Read the model definition and answer for the solid it produces. Units are mm, in the model's axes. Face numbers are marked on the shaded views. A direction names the side the tool comes from. Coordinates: 2 decimals unless noted, no trailing zeros. Write each loop counter-clockwise with the first axis right and the second up, starting at its lowest first coordinate (ties: lowest second). Pieces come first, ordered by that corner, then holes. Notation, with made-up numbers: (-19.75, -23.75) -> (-2.75, -23.75) arc R18 cw to (-2.75, -10.75) -> close; hole circle Ø11 at (76, -35.5). An arc over 180 degrees is marked (long way). Answer in a Markdown table with one row per item. Add a question column.
Item 1: Section C-C on z = 0.65 is taken. Write down the section's boundary in (x, y), then the cut area to 3 significant figures.
Item 2: Section A-A on y = 1.2 is taken. Write down the section's boundary in (x, z), then the cut area to 3 significant figures.
Item 3: Straight lines are drawn through the part: line 1 (X direction, y = 1.1, z = 2.4); line 2 (Z direction, x = -1.7, y = 3.7); line 3 (Z direction, x = -1.9, y = 1.4). For each, find the intervals that lie inside material, in ascending order. Write a range as from..to.
Item 4: Which of the six approach directions +Z, -Z, +X, -X, +Y, -Y give full straight-line access (tool end or side, diameter ignored) to the marked faces 1, 2 and 3?
Item 5: Section B-B on x = -1.55 is taken. Write down the section's boundary in (y, z).
Item 6: Section D-D on y = 4.4 is taken. Write down the section's boundary in (x, z), then the cut area to 3 significant figures.
```python
from build123d import *

# Parameters (mm, degrees)
SKETCH1_W           = 6
SKETCH1_H           = 6
BOSS_EXTRUDE1_DEPTH = 5
CUT_EXTRUDE1_DEPTH  = 2


with BuildPart() as part:
    # Sketch1 → Boss-Extrude1 (new body)
    with BuildSketch(Plane(origin=(0, 0, 0), x_dir=(1, 0, 0), z_dir=(0, 1, 0))):
        Rectangle(SKETCH1_W, SKETCH1_H)
    extrude(amount=BOSS_EXTRUDE1_DEPTH)

    # Sketch2 → Cut-Extrude1 (cut)
    with BuildSketch(Plane.ZY.offset(3)):
        Polygon((3, 5), (0, 5), (3, 2.5), align=None)
        Polygon((3, 0), (3, 2.5), (0, 0), align=None)
    extrude(amount=-CUT_EXTRUDE1_DEPTH, mode=Mode.SUBTRACT)


solid = part.part
```
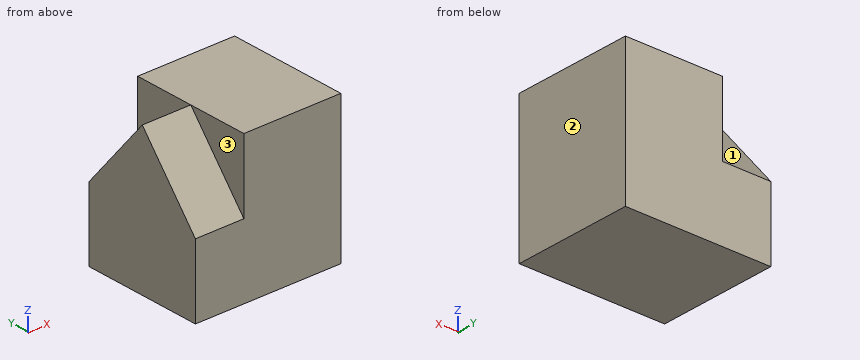
Results below:
| question | item | result |
|---|---|---|
| 1 | outline | (-3, 0.54) -> (-1, 0.54) -> (-1, 0) -> (3, 0) -> (3, 5) -> (-1, 5) -> (-1, 4.46) -> (-3, 4.46) -> close |
| 1 | area | 27.8 mm2 |
| 2 | outline | (-3, -3) -> (3, -3) -> (3, 3) -> (-1, 3) -> (-1, 1.44) -> (-3, 1.44) -> close |
| 2 | area | 32.9 mm2 |
| 3 | line 1 | x = -1..3 |
| 3 | line 2 | z = -3..1.56 |
| 3 | line 3 | z = -3..1.68 |
| 4 | face 1 | +Z, -X, +Y |
| 4 | face 2 | +Z, -Z, +X, +Y, -Y |
| 4 | face 3 | +Z, -X, -Y |
| 5 | outline | (0, -3) -> (5, -3) -> (5, 0) -> (2.5, 3) -> (0, 0) -> close |
| 6 | outline | (-3, -3) -> (3, -3) -> (3, 3) -> (-1, 3) -> (-1, 0.72) -> (-3, 0.72) -> close |
| 6 | area | 31.4 mm2 |
